Design review of the part built by this model. Coordinates are the model's own, in mm. A direction names the side the tool comes from. Coordinates: 2 decimals unless noted, no trailing zeros. Loops run counter-clockwise (first coordinate to the right, second up) from the corner with the lowest first, then second, coordinate; pieces in that order, holes last. Notation, with made-up numbers: M 20.5,-37.75 L 70.5,-37.75 A29 ccw 70.5,-5.75 Z; hole C 64.25,75 d3. An arc over 180 degrees is marked long. One line per item, written item: value.
```python
from build123d import *

# Parameters (mm, degrees)
F0_R     = 18.75
F1_DEPTH = 2.5
F3_R     = 0.5
F4_R     = 20.5
F5_DEPTH = 2
F6_D     = 4
F7_D     = 4
F8_R     = 0.5


with BuildPart() as f1:
    # F0 (on Top) → F1 (new body)
    with BuildSketch(Plane.XY):
        Circle(F0_R)
    extrude(amount=F1_DEPTH)

    # F3
    f3_edges = [f1.edges().sort_by_distance(p)[0] for p in [
        (-18.75, 0, 0),
    ]]
    fillet(f3_edges, radius=F3_R)

    # F4 (on face) → F5 (join)
    with BuildSketch(Plane.XY.offset(2.5)):
        Circle(F4_R)
    extrude(amount=F5_DEPTH)

    # F6 (through all)
    with Locations(Plane(origin=(0, 0, 2.5), x_dir=(1, 0, 0), z_dir=(0, 0, -1))):
        with Locations((-7.5, -12.990381), (-12.990381, -7.5), (-7.071068, -7.071068), (-12.990381, 7.5), (-7.071068, 7.071068), (-7.5, 12.990381), (7.5, 12.990381), (7.071068, 7.071068), (12.990381, 7.5), (7.071068, -7.071068), (7.5, -12.990381), (12.990381, -7.5)):
            Hole(F6_D / 2)

    # F7 (through all)
    with Locations(Plane.XY.offset(2.5)):
        with Locations((-12.990381, 7.5), (-7.5, 12.990381), (-7.071068, 7.071068), (-12.990381, -7.5), (-7.071068, -7.071068), (-7.5, -12.990381), (7.5, -12.990381), (7.071068, -7.071068), (12.990381, -7.5), (7.071068, 7.071068), (12.990381, 7.5), (7.5, 12.990381)):
            Hole(F7_D / 2)

    # F8
    f8_edges = [f1.edges().sort_by_distance(p)[0] for p in [
        (-20.5, 0, 2.5),
    ]]
    fillet(f8_edges, radius=F8_R)


solid = f1.part
```
(1) We need section B-B on z = 3.7. State how many separate pieces and enclosed holes the cut face has, then the cut area to 3 significant figures.
Reply:
separate pieces: 1
enclosed holes: 12
area: 1,170 mm2
(2) Tool access review of faces 1 (the cylindrical face through (9.498, 12.902, 2.282)), 2 (the cylindrical face through (-2.44, 18.59, 1.49)): name each direction out of +Z, -Z, +X, -X, +Y, -Y from which nothing blocks a thin tool from reaching the whole face with its end or side.
Reply:
face 1: +Z, -Z
face 2: -Z
(3) Mouldability with a two-part tool opening along X and no side actions: class faces 3 (the cylindrical face through (-8.146, 5.385, 2.282)), 4 (the cylindrical face through (-5.502, 12.902, 2.282)), 5 (the flat face through (6, 18, 2.5)), 6 (the cylindrical face through (-4.444, -20.013, 3.74)) as released by +X, released by -X, zero draft, split by the parting line, or undercut.
Reply:
face 3: undercut
face 4: undercut
face 5: zero draft
face 6: split by the parting line
(4) To check wall thickness, follow line 1 along Y through (x, z) = (13, 2.4); line 2 along Y through (x, z) = (7, 2.15); line 3 along Y through (x, z) = (-12.5, 4.2). State the ranges of each line that lie inside material, in increasing order. Write a range as [from, to].
Reply:
line 1: y = [-13.51, -9.5], [-5.5, 5.5], [9.5, 13.51]
line 2: y = [-17.39, -14.93], [-11.05, -9.07], [-5.07, 5.07], [9.07, 11.05], [14.93, 17.39]
line 3: y = [-16.25, -9.44], [-5.56, 5.56], [9.44, 16.25]
(5) We need section A-A on x = 0. State the section outline as (y, z) points.
Reply:
outline: M -20.5,3 A0.5 ccw -20,2.5 L -18.75,2.5 L -18.75,0.5 A0.5 ccw -18.25,0 L 18.25,0 A0.5 ccw 18.75,0.5 L 18.75,2.5 L 20,2.5 A0.5 ccw 20.5,3 L 20.5,4.5 L -20.5,4.5 Z
(6) Insertion check: pin 1 (4.5 mm diameter, centred on x = -7.5, y = -12.99, fed in from -Z); pin 2 (3 mm diameter, centred on x = 12.99, y = -7.5, fed in from -Z); pin 3 (2 mm diameter, centred on x = 9, z = 3, fed in from -Y); pin 4 (1.5 mm diameter, centred on x = 12, z = 0.5, fed in from +Y). Each pin has a flat end and moves straight along its axis. Give the tip position at first contact, or say it passes through.
Reply:
pin 1: stops at z = 0
pin 2: passes through
pin 3: stops at y = -18.87
pin 4: stops at y = 15
